For this review, take the finished solid that the model builds, in its own axes (mm). A direction names the side the tool comes from. Give positions to 0.01 mm unless a question says otherwise; leave off trailing zeros. Write each loop counter-clockwise with the first axis right and the second up, starting at its lowest first coordinate (ties: lowest second). Pieces come first, ordered by that corner, then holes. Notation, with made-up numbers: M -38.5,84.25 L 3.5,84.25 A14 cw 3.5,92.25 Z; hole C -22,83.5 d6. An arc over 180 degrees is marked long. Use one line per item in the form item = value. Start each with the question number.
Q1. For probe 1 along X at (y, z) = (0, 4.4); probe 2 along Y at (x, z) = (0.5, 1.45); probe 3 along X at (y, z) = (0, 2.4), list the stretches that pass through material, from the lowest coordinate up. Write a range as [from, to].
Q2. Consider section B-B on z = 1.8. Write out the cut boundary in (x, y), and give its area (3 significant figures).
Q3. Clearance check with flat-ended pins moving along their axes: pin 1 Ø2 at (x, y) = (-4.5, 2) entering from -Z; pin 2 Ø0.6 at (x, z) = (0.5, 4.5) entering from +Y; pin 3 Ø1.6 at (x, z) = (3.5, 5) entering from -Y; pin 4 Ø2 at (x, z) = (-4, 5.5) entering from -Y. State where each tip first meets the part, or that it passes through.
Q4. Consider section C-C on z = 3.65. Write out the cut boundary in (x, y), and give its area (3 significant figures).
Q5. Consider section A-A on y = 0. Write out the cut boundary in (x, z), and give its area (3 significant figures).
Q6. Consider section D-D on x = 3. Write out the cut boundary in (y, z), and give its area (3 significant figures).
Q7. Tool access review of faces 1 (the flat face through (0, 3, 4)), 2 (the cylindrical face through (0.867, -3.905, 0.986)), 3 (the flat face through (-0.9, -5.1, 0)): name each direction out of +Z, -Z, +X, -X, +Y, -Y from which nothing blocks a thin tool from reaching the whole face with its end or side.
Q8. Mouldability with a two-part tool opening along Y and no side actions: class faces 4 (the flat face through (-2, -1, 0)), 5 (the flat face through (2.96, -5.22, 2.96)), 6 (the flat face through (-2.96, 5.22, 2.96)), 7 (the flat face through (-3, 0, 4)) as released by +Y, released by -Y, zero draft, split by the parting line, or undercut.
```python
from build123d import *

# Parameters (mm, degrees)
ESQUISSE1_R             = 2
BASE_EXTRUSION_DEPTH    = 6
ESQUISSE2_W             = 4
ESQUISSE2_H             = 2
ESQUISSE2_W_2           = 2
ESQUISSE2_H_2           = 4
ENL_V_MAT_EXTRU_1_DEPTH = 2
ESQUISSE3_R             = 5
ESQUISSE3_R_2           = 4
ENL_V_MAT_EXTRU_2_DEPTH = 2


with BuildPart() as part:
    # Esquisse1 → Base-Extrusion (new body)
    with BuildSketch(Plane.XY):
        Polygon((0, 6.92820323), (-6, 3.464101615), (-6, -3.464101615), (0, -6.92820323), (6, -3.464101615), (6, 3.464101615), align=None)
        Circle(ESQUISSE1_R, mode=Mode.SUBTRACT)
    extrude(amount=BASE_EXTRUSION_DEPTH)

    # Esquisse2 → Enlèv. mat.-Extru.1 (cut)
    with BuildSketch(Plane.XY.offset(6)):
        Polygon((1, 1), (1, 5), (-1, 5), (-1, 1), (-1, -1), (1, -1), align=None)
        with Locations((3, 0)):
            Rectangle(ESQUISSE2_W, ESQUISSE2_H)
        with Locations((-3, 0)):
            Rectangle(ESQUISSE2_W, ESQUISSE2_H)
        with Locations((0, -3)):
            Rectangle(ESQUISSE2_W_2, ESQUISSE2_H_2)
    extrude(amount=-ENL_V_MAT_EXTRU_1_DEPTH, mode=Mode.SUBTRACT)

    # Esquisse3 → Enlèv. mat.-Extru.2 (cut)
    with BuildSketch(Plane(origin=(0, 0, 0), x_dir=(-1, 0, 0), z_dir=(0, 0, -1))):
        Circle(ESQUISSE3_R)
        Circle(ESQUISSE3_R_2, mode=Mode.SUBTRACT)
    extrude(amount=-ENL_V_MAT_EXTRU_2_DEPTH, mode=Mode.SUBTRACT)


solid = part.part
```
Working result:
q1.probe_1 = [-6, -5], [5, 6]
q1.probe_2 = [-6.64, -4.97], [-3.97, -1.94], [1.94, 3.97], [4.97, 6.64]
q1.probe_3 = [-6, -2], [2, 6]
q2.outline = M -6,-3.46 L 0,-6.93 L 6,-3.46 L 6,3.46 L 0,6.93 L -6,3.46 Z; C 0,0 d8; hole C 0,0 d10; hole C 0,0 d4
q2.area = 83.9 mm²
q3.pin_1 = 0
q3.pin_2 = 6.81
q3.pin_3 = -5.37
q3.pin_4 = -5.2
q4.outline = M -6,-3.46 L 0,-6.93 L 6,-3.46 L 6,3.46 L 0,6.93 L -6,3.46 Z; hole C 0,0 d4
q4.area = 112 mm²
q5.outline = M -6,0 L -5,0 L -5,2 L -4,2 L -4,0 L -2,0 L -2,4 L -5,4 L -5,6 L -6,6 Z; M 2,0 L 4,0 L 4,2 L 5,2 L 5,0 L 6,0 L 6,6 L 5,6 L 5,4 L 2,4 Z
q5.area = 32.0 mm²
q6.outline = M -5.2,0 L -4,0 L -4,2 L -2.65,2 L -2.65,0 L 2.65,0 L 2.65,2 L 4,2 L 4,0 L 5.2,0 L 5.2,6 L 1,6 L 1,4 L -1,4 L -1,6 L -5.2,6 Z
q6.area = 52.9 mm²
q7.face_1 = +Z
q7.face_2 = -Z
q7.face_3 = -Z, +X, -X, +Y, -Y
q8.face_4 = zero draft
q8.face_5 = released by -Y
q8.face_6 = released by +Y
q8.face_7 = undercut
